from build123d import *

# Parameters (mm, degrees)
F1_DEPTH  = 15
F2_R      = 7.5
F3_DEPTH  = 13
F4_R      = 2
F5_DEPTH  = 6
F7_DEPTH  = 3
F8_R      = 2
F9_DEPTH  = 6
F11_DEPTH = 3


with BuildPart() as f1:
    # F0 (on Front) → F1 (new body)
    with BuildSketch(Plane.XZ):
        with BuildLine():
            Line((-33.380991, 18.559887), (-103.380991, 18.559887))
            ThreePointArc((-103.380991, 18.559887), (-106.916525, 17.095421), (-108.380991, 13.559887))
            Line((-108.380991, 13.559887), (-108.380991, -36.440113))
            ThreePointArc((-108.380991, -36.440113), (-106.916525, -39.975647), (-103.380991, -41.440113))
            Line((-103.380991, -41.440113), (-33.380991, -41.440113))
            ThreePointArc((-33.380991, -41.440113), (-29.845457, -39.975647), (-28.380991, -36.440113))
            Line((-28.380991, -36.440113), (-28.380991, 13.559887))
            ThreePointArc((-28.380991, 13.559887), (-29.845457, 17.095421), (-33.380991, 18.559887))
        make_face()
    extrude(amount=F1_DEPTH)

    # F2 (on face) → F3 (cut)
    with BuildSketch(Plane.XZ.offset(15)):
        with Locations((-95.880991, 6.059887)):
            Circle(F2_R)
        with Locations((-95.880991, -28.940113)):
            Circle(F2_R)
        with Locations((-40.880991, 6.059887)):
            Circle(F2_R)
        with Locations((-40.880991, -28.940113)):
            Circle(F2_R)
    extrude(amount=-F3_DEPTH, mode=Mode.SUBTRACT)

    # F4 (on face) → F5 (cut)
    with BuildSketch(Plane.XY.offset(18.559887)):
        with Locations((-40.880991, -7.5)):
            Circle(F4_R)
        with Locations((-95.880991, -7.5)):
            Circle(F4_R)
    extrude(amount=-F5_DEPTH, mode=Mode.SUBTRACT)

    # F6 (on face) → F7 (cut)
    with BuildSketch(Plane.XY.offset(18.559887)):
        Polygon((-92.380991, -9.520726), (-92.380991, -5.479274), (-95.880991, -3.458548), (-99.380991, -5.479274), (-99.380991, -9.520726), (-95.880991, -11.541452), align=None)
        Polygon((-40.929128, -11.541165), (-37.405308, -9.56227), (-37.357171, -5.521105), (-40.832854, -3.458835), (-44.356675, -5.43773), (-44.404811, -9.478895), align=None)
    extrude(amount=-F7_DEPTH, mode=Mode.SUBTRACT)

    # F8 (on face) → F9 (cut)
    with BuildSketch(Plane(origin=(0, 0, -41.440113), x_dir=(1, 0, 0), z_dir=(0, 0, -1))):
        with Locations((-95.880991, 7.5)):
            Circle(F8_R)
        with Locations((-40.880991, 7.5)):
            Circle(F8_R)
    extrude(amount=-F9_DEPTH, mode=Mode.SUBTRACT)

    # F10 (on face) → F11 (cut)
    with BuildSketch(Plane(origin=(0, 0, -41.440113), x_dir=(1, 0, 0), z_dir=(0, 0, -1))):
        Polygon((-92.380991, 5.479274), (-92.380991, 9.520726), (-95.880991, 11.541452), (-99.380991, 9.520726), (-99.380991, 5.479274), (-95.880991, 3.458548), align=None)
        Polygon((-37.380991, 5.479274), (-37.380991, 9.520726), (-40.880991, 11.541452), (-44.380991, 9.520726), (-44.380991, 5.479274), (-40.880991, 3.458548), align=None)
    extrude(amount=-F11_DEPTH, mode=Mode.SUBTRACT)


solid = f1.part
The listing builds one solid part. Answer for the finished solid, in the listing's coordinates (mm). A direction names the side the tool comes from. Coordinates: 2 decimals unless noted, no trailing zeros. Order: outer loops, then holes, each group sorted by start corner. A loop starts at its lowest first (then second) coordinate and runs counter-clockwise, first axis right, second up. Notation, with made-up numbers: (10, 64.25) -> (49, 64.25) arc R32 cw to (49, 103.25) -> close; hole circle Ø10 at (64, 21.25). An arc over 180 degrees is marked (long way). Answer in a Markdown table with one row per item. Add a question column.
Item 1: Find section A-A (y = -10.5). Write down the section's boundary in (x, z).
Item 2: Determine the mould class of faces 1 (the face through (-69, -15, -11)), 2 (the face through (-92.381, -8, 17)), 3 (the face through (-97.655, -4.483, -39.961)) for opening direction X: +X half, -X half, draft (parallel to the pull), parting line (faces both ways), or undercut.
Item 3: Which of the six approach directions +Z, -Z, +X, -X, +Y, -Y give full straight-line access (tool end or side, diameter ignored) to faces 4 (the face through (-97.88, -7.41, 14.44)), 5 (the face through (-37.42, -8.591, -0.594)), 6 (the face through (-92.381, -7, -40))?
Item 4: Each of these flat-tipped pins is pushed along its axis until it touches: P1, Ø0.9, axis at y = -7.5, z = 18, coming from the -X side; P2, Ø7.5, axis at x = -94, z = 3, coming from the -Y side; P3, Ø3.5, axis at y = -7.5, z = 16.5, coming from the +X side. Where does it stop, or does it pass through?
Item 5: Find the intervals of material crossed by L1, parallel to Z at x = -97, y = -13.5; L2, parallel to Z at x = -46, y = -13.75; L3, parallel to X at y = -5, z = 8.5, in increasing order. Write a range as from..to.
Result set:
| question | item | result |
|---|---|---|
| 1 | outline | (-108.38, -36.44) arc R5 ccw to (-103.38, -41.44) -> (-97.68, -41.44) -> (-97.68, -38.44) -> (-94.08, -38.44) -> (-94.08, -41.44) -> (-42.68, -41.44) -> (-42.68, -38.44) -> (-39.08, -38.44) -> (-39.08, -41.44) -> (-33.38, -41.44) arc R5 ccw to (-28.38, -36.44) -> (-28.38, 13.56) arc R5 ccw to (-33.38, 18.56) -> (-39.08, 18.56) -> (-39.08, 15.56) -> (-42.68, 15.56) -> (-42.68, 18.56) -> (-94.08, 18.56) -> (-94.08, 15.56) -> (-97.68, 15.56) -> (-97.68, 18.56) -> (-103.38, 18.56) arc R5 ccw to (-108.38, 13.56) -> close; hole circle Ø15 at (-95.88, -28.94); hole circle Ø15 at (-95.88, 6.06); hole circle Ø15 at (-40.88, -28.94); hole circle Ø15 at (-40.88, 6.06) |
| 2 | face 1 | draft |
| 2 | face 2 | undercut |
| 2 | face 3 | undercut |
| 3 | face 4 | +Z |
| 3 | face 5 | -Y |
| 3 | face 6 | -Z |
| 4 | P1 | stops at x = -106.39 |
| 4 | P2 | stops at y = -2 |
| 4 | P3 | stops at x = -28.52 |
| 5 | L1 | z = -41.44..-36.36, -21.52..-1.36, 13.48..18.56 |
| 5 | L2 | z = -41.44..-34.42, -23.46..0.58, 11.54..18.56 |
| 5 | L3 | x = -108.38..-102.97, -88.79..-47.97, -33.79..-28.38 |
